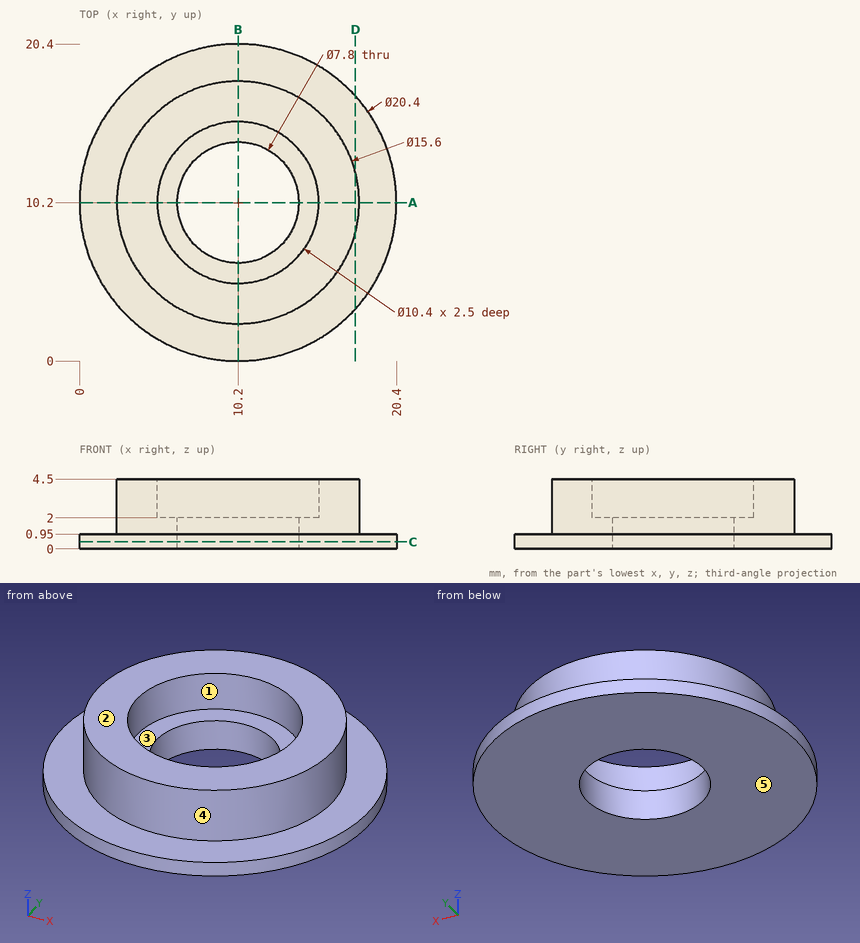
Study the drawing (mm; zero at the part's minimum x, y, z) and answer. A direction names the side the tool comes from. Coordinates: 2 decimals unless noted, no trailing zeros. Order: outer loops, then holes, each group sorted by start corner. A loop starts at its lowest first (then second) coordinate and runs counter-clockwise, first axis right, second up. Notation, with made-up numbers: M -39.75,0 L -35.75,0 A15 cw -35.75,20 Z; hole C 69.5,36.5 d1. An arc over 180 degrees is marked long. Answer as a JSON object with one key per item and string values. Group by question number.
1. Section D-D on x = 17.75 is taken. Write down the section's boundary in (y, z).
2. Flat-ended cylindrical pins translate along their axes: P1, Ø1.5, axis at y = 15.5, z = 2, coming from the -X side; P2, Ø1.5, axis at x = 14, z = 3, coming from the -Y side; P3, Ø4, axis at x = 9, y = 10.5, coming from the +Z side; P4, Ø5, axis at x = 8, y = 10, coming from the +Z side. Find the tip coordinate at first contact, or state that the pin passes through.
3. A tool of negligible diameter and unlimited length cuts with its end or side. For the marked faces 1 and 2, from which of +Z, -Z, +X, -X, +Y, -Y can it reach the whole face along a straight path? Write none if from no direction.
4. Section A-A on y = 10.2 is taken. Write down the section's boundary in (x, z).
5. Straight lines are drawn through the part: line 1 (Y direction, x = 10.2, z = 3.15); line 2 (Y direction, x = 10.2, z = 0.9); line 3 (X direction, y = 11, z = 3.95). For each, find the intervals that lie inside material, in ascending order.
6. Determine the mould class of the marked faces 3, 4 and 5 for opening direction Y: released by +Y, released by -Y, zero draft, split by the parting line, or undercut.
7. Section C-C on z = 0.45 is taken. Write down the section's boundary in (x, y), then the cut area to 3 significant figures.
Values follow:
{
 "1": {"outline": "M 3.34,0 L 17.06,0 L 17.06,0.95 L 12.16,0.95 L 12.16,4.5 L 8.24,4.5 L 8.24,0.95 L 3.34,0.95 Z"},
 "2": {"P1": "x = 3.86", "P2": "y = 3.02", "P3": "through", "P4": "z = 2"},
 "3": {"face 1": "+Z", "face 2": "+Z, +X, -X, +Y, -Y"},
 "4": {"outline": "M 0,0 L 6.3,0 L 6.3,2 L 5,2 L 5,4.5 L 2.4,4.5 L 2.4,0.95 L 0,0.95 Z; M 14.1,0 L 20.4,0 L 20.4,0.95 L 18,0.95 L 18,4.5 L 15.4,4.5 L 15.4,2 L 14.1,2 Z"},
 "5": {"line 1": "2.4 to 5, 15.4 to 18", "line 2": "0 to 6.3, 14.1 to 20.4", "line 3": "2.44 to 5.06, 15.34 to 17.96"},
 "6": {"face 3": "undercut", "face 4": "split by the parting line", "face 5": "zero draft"},
 "7": {"outline": "C 10.2,10.2 d20.4; hole C 10.2,10.2 d7.8", "area": "279 mm2"}
}
